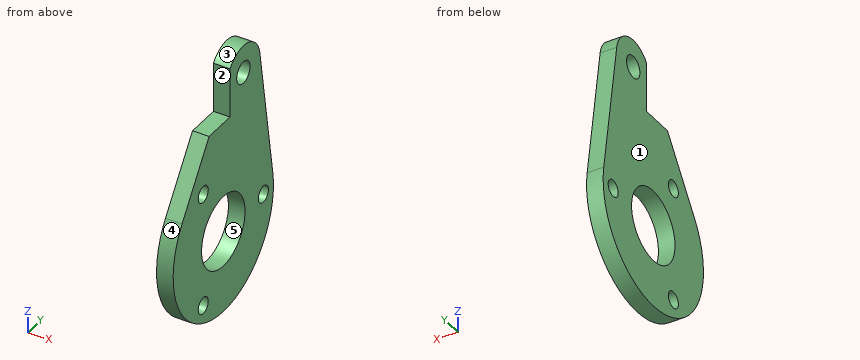
```python
from build123d import *

# Parameters (mm, degrees)
ESQUISSE1_R             = 6.5
ESQUISSE1_R_2           = 1.5
ESQUISSE1_R_3           = 2
BOSS_EXTRU_1_DEPTH      = 3
ENL_V_MAT_EXTRU_1_DEPTH = 4


with BuildPart() as part:
    # Esquisse1 → Boss.-Extru.1 (new body)
    with BuildSketch(Plane.ZY):
        with BuildLine():
            Line((29.049319561, 1.891304582), (8.547958684, -12.326086254))
            ThreePointArc((8.547958684, -12.326086254), (-14.621490903, -3.348433031), (2.331837562, 14.817642646))
            Line((2.331837562, 14.817642646), (26.977279187, 10.939214215))
            ThreePointArc((26.977279187, 10.939214215), (31.073830301, 7.116144344), (29.049319561, 1.891304582))
        make_face()
        Circle(ESQUISSE1_R, mode=Mode.SUBTRACT)
        with Locations((-10.392304845, -6)):
            Circle(ESQUISSE1_R_2, mode=Mode.SUBTRACT)
        with Locations((0, 12)):
            Circle(ESQUISSE1_R_2, mode=Mode.SUBTRACT)
        with Locations((10.392304845, -6)):
            Circle(ESQUISSE1_R_2, mode=Mode.SUBTRACT)
        with Locations((26.2, 6)):
            Circle(ESQUISSE1_R_3, mode=Mode.SUBTRACT)
    extrude(amount=-BOSS_EXTRU_1_DEPTH)

    # Esquisse2 → Enlèv. mat.-Extru.1 (cut, through all)
    with BuildSketch(Plane(origin=(3, 0, 0), x_dir=(0, 0, -1), z_dir=(1, 0, 0))):
        Polygon((-29.206057462, 2), (-20.2, 2), (-20.2, -4.245567774), align=None)
    extrude(amount=-ENL_V_MAT_EXTRU_1_DEPTH, mode=Mode.SUBTRACT)


solid = part.part
```
Source: CAD feature listing. Evaluate the final solid. Frame: model axes, mm. Face numbers are marked on the shaded views. A direction names the side the tool comes from. Coordinates: 2 decimals unless noted, no trailing zeros. Order: outer loops, then holes, each group sorted by start corner. A loop starts at its lowest first (then second) coordinate and runs counter-clockwise, first axis right, second up. Notation, with made-up numbers: (-27, 82) - (-13, 82) arc R11 ccw to (-13, 96) - close; hole circle Ø6 at (26.5, 16.5). An arc over 180 degrees is marked (long way). One line per item, written item: value.
1) Cut plane A-A on y = 0. Output: boundary loops of the cut face in (x, z), plus the area to 3 significant figures.
Computed values:
outline: (0, -15) - (3, -15) - (3, -6.5) - (0, -6.5) - close; (0, 6.5) - (3, 6.5) - (3, 20.2) - (0, 20.2) - close
area: 66.6 mm^2
2) Reachability of the marked faces 1 and 2 from +Z, -Z, +X, -X, +Y, -Y: full face, straight path, thin tool, end or side. Return the list, or none.
Computed values:
face 1: +Z, -Z, -X, +Y, -Y
face 2: +Z, +X, -X, -Y
3) Mould query, pull axis Z, two halves, no side actions, for the marked faces 3, 4 and 5. Classes: released by +Z, released by -Z, zero draft, split by the parting line, or undercut.
Computed values:
face 3: released by +Z
face 4: split by the parting line
face 5: undercut
4) Cut plane C-C on x = 1.6. Output: boundary loops of the cut face in (y, z).
Computed values:
outline: (-12.33, 8.55) arc R15 ccw (long way) to (14.82, 2.33) - (10.94, 26.98) arc R5 ccw to (2, 29.2) - (2, 20.2) - (-4.25, 20.2) - close; hole circle Ø3 at (-6, -10.39); hole circle Ø3 at (-6, 10.39); hole circle Ø13 at (0, 0); hole circle Ø4 at (6, 26.2); hole circle Ø3 at (12, 0)
5) Cut plane B-B on z = 0. Output: boundary loops of the cut face in (x, y).
Computed values:
outline: (0, -15) - (3, -15) - (3, -6.5) - (0, -6.5) - close; (0, 6.5) - (3, 6.5) - (3, 10.5) - (0, 10.5) - close; (0, 13.5) - (3, 13.5) - (3, 15) - (0, 15) - close
6) Ray query, line 1 (Z direction, x = 2.3, y = -5.5); line 2 (Y direction, x = 0.5, z = -0.5); line 3 (Y direction, x = 2.2, z = 27). Return the intervals inside material, ascending. Write a range as [from, to].
Computed values:
line 1: z = [-13.96, -11.81], [-8.98, -3.46], [3.46, 8.98], [11.81, 18.39]
line 2: y = [-14.99, -6.48], [6.48, 10.59], [13.41, 14.99]
line 3: y = [2, 4.17], [7.83, 10.94]
7) Contact query for flat-ended pins moving along their axis: pin 1 (1.8 mm diameter, centred on y = -6, z = 10.39, fed in from +X); pin 2 (1.5 mm diameter, centred on x = 2.5, y = 4.5, fed in from +Z). Output: stop coordinate, or through.
Computed values:
pin 1: passes through
pin 2: stops at z = 31.14
8) Cut plane D-D on z = -9.5. Output: boundary loops of the cut face in (x, y), plus the area to 3 significant figures.
Computed values:
outline: (0, -11.61) - (3, -11.61) - (3, -7.21) - (0, -7.21) - close; (0, -4.79) - (3, -4.79) - (3, 11.61) - (0, 11.61) - close
area: 62.4 mm^2
